```python
from build123d import *

# Parameters (mm, degrees)
BASE_FLANGE1_DEPTH      = 146.05
EDGE_FLANGE1_DEPTH      = 189.0268
SKETCH9_R               = 3.175
CUT_EXTRUDE1_DEPTH      = 210.261164577
CUT_EXTRUDE2_DEPTH      = 208.932201991
CUT_EXTRUDE2_DEPTH_BACK = 208.932201991
TAB1_START              = -3.175
SKETCH15_R              = 9.525
SKETCH15_R_2            = 3.175
TAB1_DEPTH              = 3.175


# Sheet-metal steps are written as plain solids
with BuildPart() as part:
    # Sketch1 → Base-Flange1 (new body)
    with BuildSketch(Plane.XY):
        with BuildLine():
            Line((120.65, 85.725), (99.1616, 85.725))
            ThreePointArc((99.1616, 85.725), (96.395681115, 84.579318885), (95.25, 81.8134))
            Line((95.25, 81.8134), (95.25, 0.7366))
            ThreePointArc((95.25, 0.7366), (95.034254855, 0.215745145), (94.5134, 0))
            Line((94.5134, 0), (-94.5134, 0))
            ThreePointArc((-94.5134, 0), (-95.034254855, 0.215745145), (-95.25, 0.7366))
            Line((-95.25, 0.7366), (-95.25, 81.8134))
            ThreePointArc((-95.25, 81.8134), (-96.395681115, 84.579318885), (-99.1616, 85.725))
            Line((-99.1616, 85.725), (-120.65, 85.725))
            Line((-120.65, 85.725), (-120.65, 82.55))
            Line((-120.65, 82.55), (-99.1616, 82.55))
            ThreePointArc((-99.1616, 82.55), (-98.640745145, 82.334254855), (-98.425, 81.8134))
            Line((-98.425, 81.8134), (-98.425, 0.7366))
            ThreePointArc((-98.425, 0.7366), (-97.279318885, -2.029318885), (-94.5134, -3.175))
            Line((-94.5134, -3.175), (94.5134, -3.175))
            ThreePointArc((94.5134, -3.175), (97.279318885, -2.029318885), (98.425, 0.7366))
            Line((98.425, 0.7366), (98.425, 81.8134))
            ThreePointArc((98.425, 81.8134), (98.640745145, 82.334254855), (99.1616, 82.55))
            Line((99.1616, 82.55), (120.65, 82.55))
            Line((120.65, 82.55), (120.65, 85.725))
        make_face()
    extrude(amount=BASE_FLANGE1_DEPTH)

    # Edge-Flange1 section (across the edge) → Edge-Flange1 (add)
    with BuildSketch(Plane(origin=(94.5134, 0, -0.7366), x_dir=(0, 0, 1), z_dir=(-1, 0, 0))):
        with BuildLine():
            Line((-3.175, 0.7366), (-3.175, 22.225))
            Line((-3.175, 22.225), (0, 22.225))
            Line((0, 22.225), (0, 0.7366))
            ThreePointArc((0, 0.7366), (0.215745145, 0.215745145), (0.7366, 0))
            Line((0.7366, 0), (0.7366, -3.175))
            ThreePointArc((0.7366, -3.175), (-2.029318885, -2.029318885), (-3.175, 0.7366))
        make_face()
    extrude(amount=EDGE_FLANGE1_DEPTH)

    # Sketch9 → Cut-Extrude1 (cut, through all)
    with BuildSketch(Plane(origin=(0, 85.725, 0), x_dir=(1, 0, 0), z_dir=(0, 1, 0))):
        with Locations(Location((-114.3, -19.05, 0), (0, 0, 180))):
            Circle(SKETCH9_R)
        with Locations(Location((-107.95, -73.025, 0), (0, 0, 180))):
            Circle(SKETCH9_R)
        with Locations(Location((-107.95, -133.35, 0), (0, 0, 180))):
            Circle(SKETCH9_R)
        with Locations(Location((107.95, -133.35, 0), (0, 0, 180))):
            Circle(SKETCH9_R)
        with Locations(Location((107.95, -73.025, 0), (0, 0, 180))):
            Circle(SKETCH9_R)
        with Locations(Location((107.95, -12.7, 0), (0, 0, 180))):
            Circle(SKETCH9_R)
    extrude(amount=-CUT_EXTRUDE1_DEPTH, mode=Mode.SUBTRACT)

    # Sketch14 → Cut-Extrude2 (cut, two sides: drawn at the far end of the back side and taken through both)
    with BuildSketch(Plane(origin=(0, 0, 0), x_dir=(0, 1, 0), z_dir=(-1, 0, 0)).offset(-CUT_EXTRUDE2_DEPTH_BACK)):
        with BuildLine():
            Line((42.0116, -127), (13.4366, -127))
            ThreePointArc((13.4366, -127), (11.8491, -125.4125), (13.4366, -123.825))
            Line((13.4366, -123.825), (42.0116, -123.825))
            ThreePointArc((42.0116, -123.825), (43.5991, -125.4125), (42.0116, -127))
        make_face()
    extrude(amount=CUT_EXTRUDE2_DEPTH + CUT_EXTRUDE2_DEPTH_BACK, mode=Mode.SUBTRACT)

    # Sketch15 → Tab1 (add)
    with BuildSketch(Plane.XZ.offset(-82.55).offset(TAB1_START)):
        with Locations((-114.3, 19.05)):
            Circle(SKETCH15_R)
        with Locations(Location((-114.3, 19.05, 0), (0, 0, 180))):
            Circle(SKETCH15_R_2, mode=Mode.SUBTRACT)
    extrude(amount=TAB1_DEPTH)


solid = part.part
```
For this review, take the finished solid that the model builds, in its own axes (mm). A direction names the side the tool comes from. Coordinates: 2 decimals unless noted, no trailing zeros. Loops run counter-clockwise (first coordinate to the right, second up) from the corner with the lowest first, then second, coordinate; pieces in that order, holes last. Notation, with made-up numbers: (-20.5, -21.75) - (14.5, -21.75) arc R18 ccw to (14.5, 13.25) - close; hole circle Ø8 at (28.25, 37.5). An arc over 180 degrees is marked (long way). Use one line per item in the form item = value. Start each with the question number.
1) Take a section at A-A (z = 19.05). State the section outline as (x, y) points (3 decimals), plus the area to 3 significant figures.
2) Take a section at C-C (y = 78). State the section outline as (x, z) points (3 decimals).
3) Draft analysis for pull direction Z (two halves, no side actions). For faces 5 (the face through (98, 51, 0)), 6 (the face through (-112, 82.55, 72)), 7 (the face through (-107.262, 84.16, 69.926)), state which applies: released by +Z, released by -Z, zero draft, split by the parting line, or undercut.
4) For pin 1 (10.5 mm diameter, centred on x = 16, y = 13, fed in from +Z); pin 2 (3.5 mm diameter, centred on y = 84, z = 6.5, fed in from -X); pin 3 (8 mm diameter, centred on y = 27, z = 74.5, fed in from -X) (3 decimals), all flat-tipped, find the tip position at first contact; note any pin that passes through.
5) Take a section at D-D (x = -114.3). State the section outline as (y, z) points (3 decimals), plus the area to 3 significant figures.
6) For faces 1 (the face through (1, 12, -0.737)), 2 (the face through (-98.425, 42, 72)), 3 (the face through (95.25, 42, 72)), 4 (the face through (98.425, 41, 72)), list the 3-axis set-ups (+Z, -Z, +X, -X, +Y, -Y) from which the entire face can be reached by the end or side of a thin tool; tool diameter is ignored.
7) To check wall thickness, follow probe 1 along Z at (x, y) = (107.95, 83.55) (3 decimals); probe 2 along Z at (x, y) = (-107.95, 83.9) (3 decimals); probe 3 along Z at (x, y) = (107, 83). State the ranges of each line that lie inside material, in increasing order. Write a range as from..to.
8) Take a section at B-B (x = 107.95). State the section outline as (y, z) points (3 decimals).
From the geometry:
q1.outline = (-123.825, 82.55) - (-117.475, 82.55) - (-117.475, 85.725) - (-123.825, 85.725) - close; (-111.125, 82.55) - (-99.162, 82.55) arc R0.737 cw to (-98.425, 81.813) - (-98.425, 0.737) arc R3.912 ccw to (-94.513, -3.175) - (94.513, -3.175) arc R3.912 ccw to (98.425, 0.737) - (98.425, 81.813) arc R0.737 cw to (99.162, 82.55) - (120.65, 82.55) - (120.65, 85.725) - (99.162, 85.725) arc R3.912 ccw to (95.25, 81.813) - (95.25, 0.737) arc R0.737 cw to (94.513, 0) - (-94.513, 0) arc R0.737 cw to (-95.25, 0.737) - (-95.25, 81.813) arc R3.912 ccw to (-99.162, 85.725) - (-111.125, 85.725) - close
q1.area = 1,290 mm2
q2.outline = (-98.425, 0) - (-95.25, 0) - (-95.25, 146.05) - (-98.425, 146.05) - close; (95.25, 0) - (98.425, 0) - (98.425, 146.05) - (95.25, 146.05) - close
q3.face_5 = released by -Z
q3.face_6 = zero draft
q3.face_7 = undercut
q4.pin_1 = -0.74
q4.pin_2 = -120.65
q4.pin_3 = -98.425
q5.outline = (82.55, 0) - (85.725, 0) - (85.725, 15.875) - (82.55, 15.875) - close; (82.55, 22.225) - (85.725, 22.225) - (85.725, 146.05) - (82.55, 146.05) - close
q5.area = 444 mm2
q6.face_1 = +Z, +X, -X, +Y
q6.face_2 = +Z, -Z, -X, -Y
q6.face_3 = +Z, -Z, +Y
q6.face_4 = +Z, -Z, +X, -Y
q7.probe_1 = 0..9.525, 15.875..69.85, 76.2..130.175, 136.525..146.05
q7.probe_2 = 0..69.85, 76.2..130.175, 136.525..146.05
q7.probe_3 = 0..9.67, 15.73..70, 76.05..130.32, 136.38..146.05
q8.outline = (82.55, 0) - (85.725, 0) - (85.725, 9.525) - (82.55, 9.525) - close; (82.55, 15.875) - (85.725, 15.875) - (85.725, 69.85) - (82.55, 69.85) - close; (82.55, 76.2) - (85.725, 76.2) - (85.725, 130.175) - (82.55, 130.175) - close; (82.55, 136.525) - (85.725, 136.525) - (85.725, 146.05) - (82.55, 146.05) - close
